from build123d import *

# Parameters (mm, degrees)
SKETCH1_W               = 38
SKETCH1_H               = 27.5
BOSS_EXTRUDE1_DEPTH     = 7
SKETCH2_W               = 36
SKETCH2_H               = 25.5
CUT_EXTRUDE1_DEPTH      = 3
SKETCH3_RX              = 16.007748615
SKETCH3_RY              = 10.755206101
CUT_EXTRUDE2_DEPTH      = 4
CUT_EXTRUDE2_DEPTH_BACK = 5
CUT_EXTRUDE4_DEPTH      = 1.5
CUT_EXTRUDE5_DEPTH      = 14.7500001
CUT_EXTRUDE5_DEPTH_BACK = 14.7500001


with BuildPart() as part:
    # Sketch1 → Boss-Extrude1 (new body)
    with BuildSketch(Plane(origin=(0, 0, 0), x_dir=(1, 0, 0), z_dir=(0, 1, 0))):
        Rectangle(SKETCH1_W, SKETCH1_H)
    extrude(amount=-BOSS_EXTRUDE1_DEPTH)

    # Sketch2 → Cut-Extrude1 (cut)
    with BuildSketch(Plane(origin=(0, 0, 0), x_dir=(1, 0, 0), z_dir=(0, 1, 0))):
        Rectangle(SKETCH2_W, SKETCH2_H)
    extrude(amount=-CUT_EXTRUDE1_DEPTH, mode=Mode.SUBTRACT)

    # Sketch3 → Cut-Extrude2 (cut, two sides)
    with BuildSketch(Plane(origin=(0, -3, 0), x_dir=(1, 0, 0), z_dir=(0, 1, 0))) as cut_extrude2_sk:
        with Locations(Location((0, 0), (0, 0, -1.782797699))):
            Ellipse(SKETCH3_RX, SKETCH3_RY)
    extrude(amount=CUT_EXTRUDE2_DEPTH, mode=Mode.SUBTRACT)
    extrude(cut_extrude2_sk.sketch, amount=-CUT_EXTRUDE2_DEPTH_BACK, mode=Mode.SUBTRACT)

    # Sketch8 → Cut-Extrude4 (cut, symmetric)
    with BuildSketch(Plane(origin=(0, -5, 0), x_dir=(-1, 0, 0), z_dir=(0, -1, 0))):
        with BuildLine():
            Line((-14.5, 11), (-14.5, 23.562662058))
            Line((-14.5, 23.562662058), (-9.5, 23.562662058))
            Line((-9.5, 23.562662058), (-9.5, 11))
            ThreePointArc((-9.5, 11), (-12, 8.5), (-14.5, 11))
        make_face()
        with BuildLine():
            Line((9.5, 23.562662058), (9.5, 11))
            ThreePointArc((9.5, 11), (12, 8.5), (14.5, 11))
            Line((14.5, 11), (14.5, 23.562662058))
            Line((14.5, 23.562662058), (9.5, 23.562662058))
        make_face()
        with BuildLine():
            Line((14.5, -11), (14.5, -23.562662058))
            Line((14.5, -23.562662058), (9.5, -23.562662058))
            Line((9.5, -23.562662058), (9.5, -11))
            ThreePointArc((9.5, -11), (12, -8.5), (14.5, -11))
        make_face()
        with BuildLine():
            Line((-9.5, -23.562662058), (-9.5, -11))
            ThreePointArc((-9.5, -11), (-12, -8.5), (-14.5, -11))
            Line((-14.5, -11), (-14.5, -23.562662058))
            Line((-14.5, -23.562662058), (-9.5, -23.562662058))
        make_face()
    extrude(amount=CUT_EXTRUDE4_DEPTH, both=True, mode=Mode.SUBTRACT)

    # Sketch9 → Cut-Extrude5 (cut, two sides)
    with BuildSketch(Plane.XY) as cut_extrude5_sk:
        Polygon((-15.498962309, -7), (-19, -2), (-19, -7), align=None)
        Polygon((19, -7), (15.498962309, -7), (19, -2), align=None)
    extrude(amount=CUT_EXTRUDE5_DEPTH, mode=Mode.SUBTRACT)
    extrude(cut_extrude5_sk.sketch, amount=-CUT_EXTRUDE5_DEPTH_BACK, mode=Mode.SUBTRACT)


solid = part.part
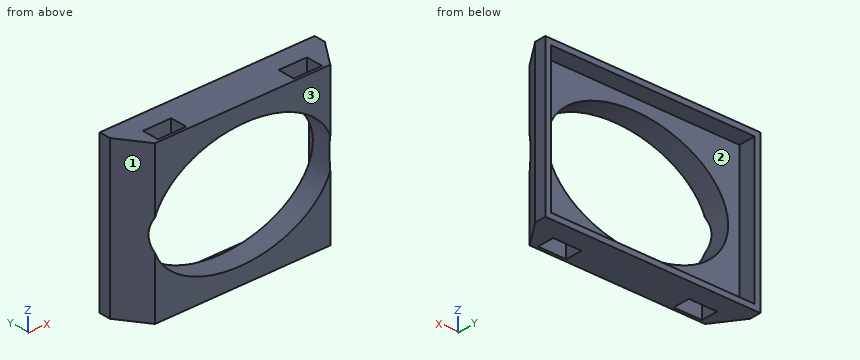
Check sheet for the modelled part. Datum: model origin and axes. Units: mm. Face numbers are marked on the shaded views. Coordinates: 2 decimals unless noted, no trailing zeros. Loops run counter-clockwise (first coordinate to the right, second up) from the corner with the lowest first, then second, coordinate; pieces in that order, holes last. Notation, with made-up numbers: (64, 40) -> (96, 40) arc R21 ccw to (96, 72) -> close; hole circle Ø6 at (65.5, 82). An arc over 180 degrees is marked (long way). Write item = value, one per line. Start each with the question number.
1. Depth check by flat-ended pin: P1, Ø0.8, axis at y = -5, z = 13, coming from the +X side; P2, Ø2, axis at y = -4.5, z = -12, coming from the -X side; P3, Ø3, axis at y = -5.5, z = -13, coming from the +X side. Enter the tip coordinate at first touch or a pass-through.
2. Section check A-A on y = -1.5. Record the cut outline in (x, z).
3. Material ranges on line 1 (Z direction, x = -2, y = -2.5); line 2 (X direction, y = -2, z = 6.5); line 3 (X direction, y = -6, z = 12.75), recorded low to high.
4. Draft check along X on the marked faces 1, 2 and 3. Enter one of: released by +X, released by -X, zero draft, split by the parting line, or undercut.
5. Section check B-B on z = -10. Give the number of separate pieces and of enclosed holes in the cut face, then the cut area to 3 significant figures.
Responses:
q1.P1 = 17.18
q1.P2 = -17.95
q1.P3 = 17.6
q2.outline = (-19, -13.75) -> (19, -13.75) -> (19, 13.75) -> (-19, 13.75) -> close; hole (-18, -12.75) -> (18, -12.75) -> (18, 12.75) -> (-18, 12.75) -> close
q3.line_1 = -13.75 to -12.75, 12.75 to 13.75
q3.line_2 = -19 to -18, 18 to 19
q3.line_3 = -16.2 to -14.5, -9.5 to 9.5, 14.5 to 16.2
q4.face_1 = released by -X
q4.face_2 = undercut
q4.face_3 = zero draft
q5.separate_pieces = 2
q5.enclosed_holes = 2
q5.area = 65.7 mm2
